Part print with two shaded views. Sizes in mm from the minimum x, y, z corner. Round coordinates to 2 decimals unless told otherwise and drop trailing zeros. Order: outer loops, then holes, each group sorted by start corner. A loop starts at its lowest first (then second) coordinate and runs counter-clockwise, first axis right, second up. Notation, with made-up numbers: M 0.25,-8.75 L 45.25,-8.75 A21 ccw 45.25,9.25 Z; hole C -17.5,-36 d8. An arc over 180 degrees is marked long. Put each result on its own line as item: value.
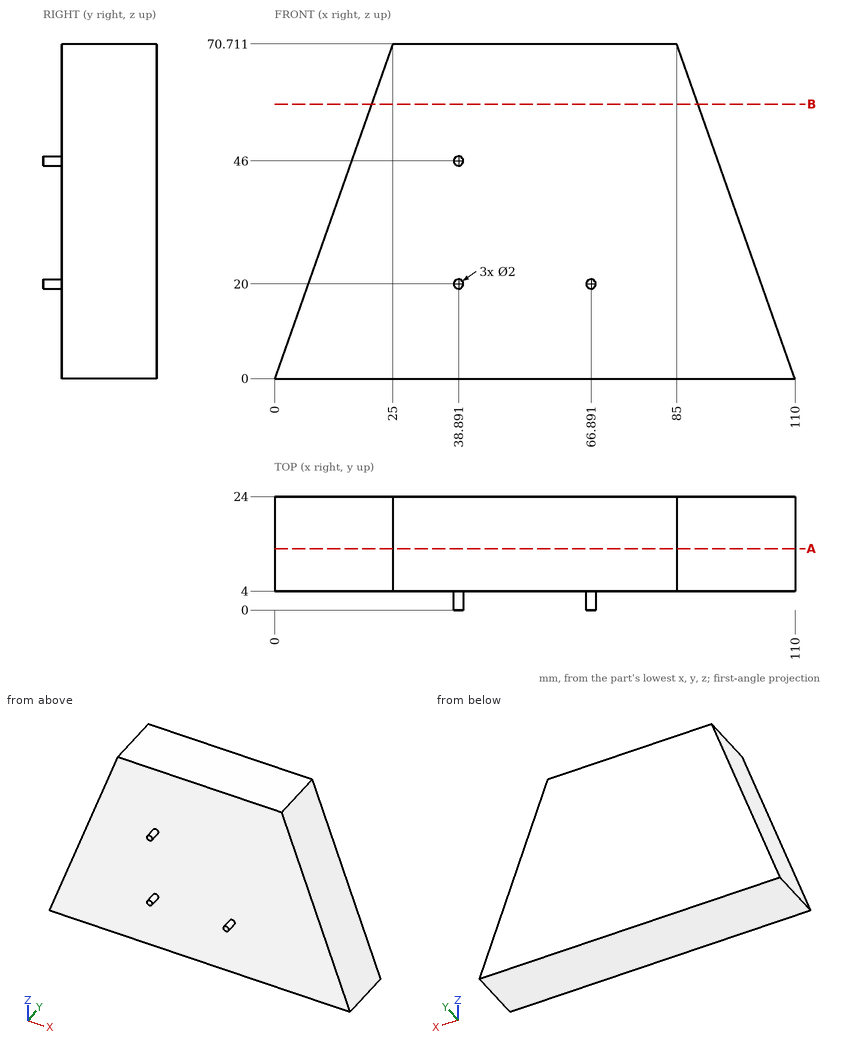
Item 1: Pin check, flat tips, straight feed: P1, Ø3, axis at y = 5, z = 55.5, coming from the -X side; P2, Ø1.5, axis at x = 77, z = 34, coming from the -Y side; P3, Ø12, axis at y = 8.5, z = 33, coming from the +X side. Stop position of each tip, or through.
Answers below:
P1: x = 19.09
P2: y = 4
P3: x = 100.45
Item 2: Probe line 1 along Y through (x, z) = (94, 27); line 2 along X through (y, z) = (15.25, 41) (1 decimal); line 3 along X through (y, z) = (15.25, 55.5). List the from-to ranges inside material, lowest first. Write a range as [from, to].
Answers below:
line 1: [4, 24]
line 2: [14.5, 95.5]
line 3: [19.62, 90.38]
Item 3: Band-saw the part on A-A on y = 13. Give the cut face in (x, z), and give its area (3 significant figures).
Answers below:
outline: M 0,0 L 110,0 L 85,70.71 L 25,70.71 Z
area: 6,010 mm²
Item 4: Band-saw the part on B-B on z = 58. Give the cut face in (x, y), and give its area (3 significant figures).
Answers below:
outline: M 20.51,4 L 89.49,4 L 89.49,24 L 20.51,24 Z
area: 1,380 mm²
